from build123d import *

# Parameters (mm, degrees)
EXTRUDE_1_DEPTH     = 20
SKETCH_2_R          = 3
CUT_EXTRUDE_1_DEPTH = 21.25


with BuildPart() as part:
    # 草图1 → 凸台-拉伸1 (new body)
    with BuildSketch(Plane.XY):
        with BuildLine():
            Line((-33.25, 0), (-18.25, 0))
            ThreePointArc((-18.25, 0), (0, 18.25), (18.25, 0))
            Line((18.25, 0), (33.25, 0))
            Line((33.25, 0), (33.25, 20.25))
            Line((33.25, 20.25), (-33.25, 20.25))
            Line((-33.25, 20.25), (-33.25, 0))
        make_face()
    extrude(amount=EXTRUDE_1_DEPTH)

    # 草图2 → 切除-拉伸1 (cut, through all)
    with BuildSketch(Plane(origin=(0, 20.25, 0), x_dir=(1, 0, 0), z_dir=(0, 1, 0))):
        with Locations((-25.5, -10)):
            Circle(SKETCH_2_R)
        with Locations((25.5, -10)):
            Circle(SKETCH_2_R)
    extrude(amount=-CUT_EXTRUDE_1_DEPTH, mode=Mode.SUBTRACT)


solid = part.part
Here's how the part is built. I have some questions about the finished solid (model axes, mm). Round coordinates to 2 decimals unless told otherwise and drop trailing zeros. Loops run counter-clockwise (first coordinate to the right, second up) from the corner with the lowest first, then second, coordinate; pieces in that order, holes last.
1. If I drill on line 1 along Z through (x, y) = (-25.5, 5.5); line 2 along X through (y, z) = (10.25, 11); line 3 along X through (y, z) = (14.5, 10), over which ranges is the centre line in solid material (lowest first)?
Answer list:
line 1: z = 0 to 7, 13 to 20
line 2: x = -33.25 to -28.33, -22.67 to -15.1, 15.1 to 22.67, 28.33 to 33.25
line 3: x = -33.25 to -28.5, -22.5 to -11.08, 11.08 to 22.5, 28.5 to 33.25
2. If we section it at A-A on z = 10: Write out the boundary of the cut face in (x, y).
Answer list:
outline: (-33.25, 0) - (-28.5, 0) - (-28.5, 20.25) - (-33.25, 20.25) - close; (-22.5, 0) - (-18.25, 0) arc R18.25 cw to (18.25, 0) - (22.5, 0) - (22.5, 20.25) - (-22.5, 20.25) - close; (28.5, 0) - (33.25, 0) - (33.25, 20.25) - (28.5, 20.25) - close
3. We'd pull the mould along Z, two halves only. Please class faces 1 (the face through (33.25, 10, 10)), 2 (the face through (0, 19, 0)), 3 (the face through (25.109, 10.267, 7.026)), 4 (the face through (-28.5, 10.3, 9.9)): +Z half, -Z half, draft (parallel to the pull), parting line (faces both ways), or undercut.
Answer list:
face 1: draft
face 2: -Z half
face 3: undercut
face 4: undercut
4. For P1, Ø7, axis at x = -25.5, z = 10, coming from the -Y side; P2, Ø5, axis at x = 25.5, z = 10, coming from the +Y side; P3, Ø1.5, axis at x = -8.5, z = 10, coming from the -Y side, each with a flat end and sliding along its axis, tell me the tip position at first contact or that it passes through.
Answer list:
P1: stops at y = 0
P2: passes through
P3: stops at y = 15.73
5. If we section it at D-D on y = 2: Write out the boundary of the cut face in (x, z), plus the area to 3 significant figures.
Answer list:
outline: (-33.25, 0) - (-18.14, 0) - (-18.14, 20) - (-33.25, 20) - close; (18.14, 0) - (33.25, 0) - (33.25, 20) - (18.14, 20) - close; hole circle Ø6 at (-25.5, 10); hole circle Ø6 at (25.5, 10)
area: 548 mm2
6. If we section it at C-C on x = 25.5: Write out the boundary of the cut face in (y, z).
Answer list:
outline: (0, 0) - (20.25, 0) - (20.25, 7) - (0, 7) - close; (0, 13) - (20.25, 13) - (20.25, 20) - (0, 20) - close
7. If we section it at B-B on y = 7: Write out the boundary of the cut face in (x, z), plus the area to 3 significant figures.
Answer list:
outline: (-33.25, 0) - (-16.85, 0) - (-16.85, 20) - (-33.25, 20) - close; (16.85, 0) - (33.25, 0) - (33.25, 20) - (16.85, 20) - close; hole circle Ø6 at (-25.5, 10); hole circle Ø6 at (25.5, 10)
area: 599 mm2
